Answer from the drawing. Dimensions are ordinates in mm from the lowest x, y and z of the part. Coordinates: 2 decimals unless noted, no trailing zeros. Write each loop counter-clockwise with the first axis right and the second up, starting at its lowest first coordinate (ties: lowest second). Pieces come first, ordered by that corner, then holes. Notation, with made-up numbers: (11, 5) - (33, 5) arc R5 ccw to (33, 11) - close; hole circle Ø7 at (36, -35.75). An arc over 180 degrees is marked (long way). Answer as a JSON object with one key per item and string values. Group by question number.
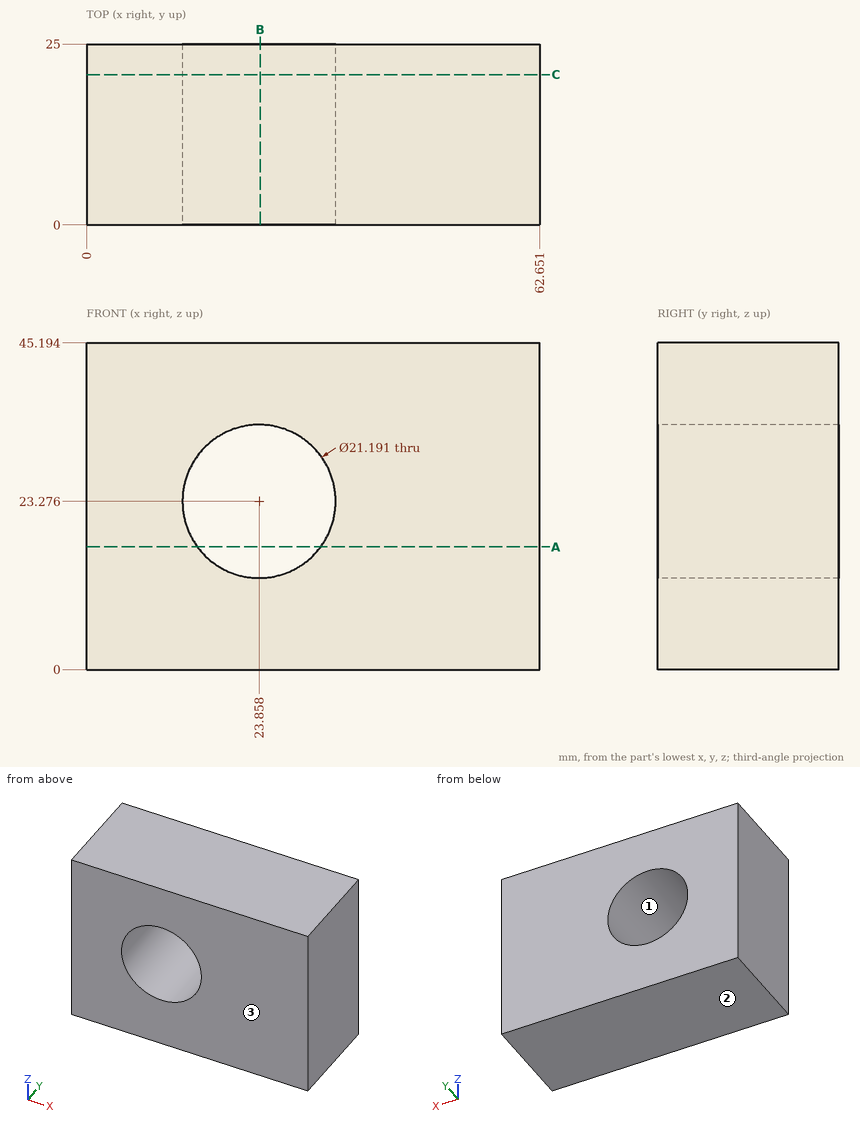
Q1. For a pull along Z with two mould halves and no side action, classify the marked faces 1, 2 and 3 as +Z half, -Z half, draft (parallel to the pull), parting line (faces both ways), or undercut.
Q2. Section C-C on y = 20.75 is taken. Determine the outline of the cut face in (x, z), plus the area to 3 significant figures.
Q3. Section A-A on z = 17 is taken. Determine the outline of the cut face in (x, y) (1 decimal).
Q4. Section B-B on x = 24 is taken. Determine the outline of the cut face in (y, z), plus the area to 3 significant figures.
Q5. Consider L1, parallel to X at y = 7.5, z = 18; L2, parallel to X at y = 6.75, z = 20; L3, parallel to Z at x = 22, y = 21.25 (1 decimal). Determine where each line is inside the solid, lowest interval first. Write a range as from..to.
Numbers:
{
 "1": {"face 1": "undercut", "face 2": "-Z half", "face 3": "draft"},
 "2": {"outline": "(0, 0) - (62.65, 0) - (62.65, 45.19) - (0, 45.19) - close; hole circle Ø21.19 at (23.86, 23.28)", "area": "2,480 mm²"},
 "3": {"outline": "(0, 0) - (15.3, 0) - (15.3, 25) - (0, 25) - close; (32.4, 0) - (62.7, 0) - (62.7, 25) - (32.4, 25) - close"},
 "4": {"outline": "(0, 0) - (25, 0) - (25, 12.68) - (0, 12.68) - close; (0, 33.87) - (25, 33.87) - (25, 45.19) - (0, 45.19) - close", "area": "600 mm²"},
 "5": {"L1": "x = 0..14.67, 33.05..62.65", "L2": "x = 0..13.78, 33.93..62.65", "L3": "z = 0..12.8, 33.7..45.2"}
}
